Source: three-view drawing plus pictorial views. Frame: mm from the lowest corner of the part. A direction names the side the tool comes from. Give positions to 0.01 mm unless a question says otherwise; leave off trailing zeros. Write each loop counter-clockwise with the first axis right and the second up, starting at its lowest first coordinate (ties: lowest second). Pieces come first, ordered by that corner, then holes.
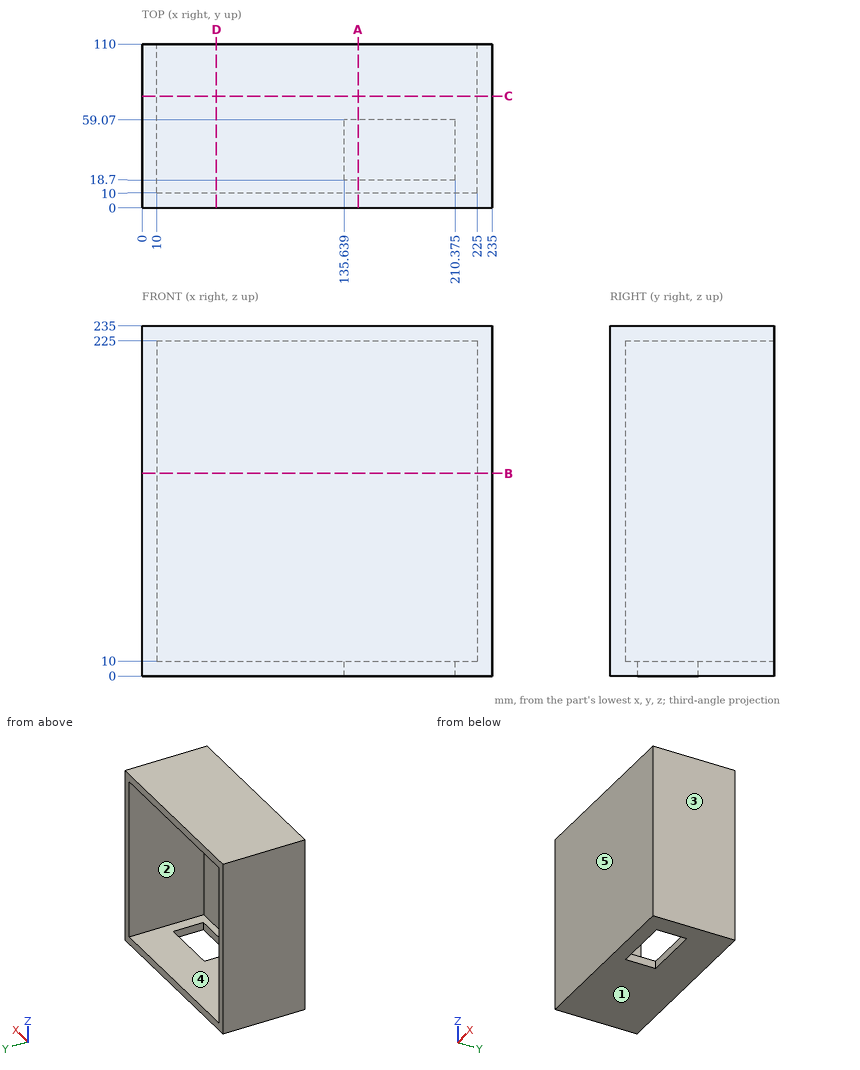
Q1. Section B-B on z = 136. Output: boundary loops of the cut face in (x, y).
Filled sheet:
outline: (0, 0) - (235, 0) - (235, 110) - (225, 110) - (225, 10) - (10, 10) - (10, 110) - (0, 110) - close
Q2. Pin query (flat end, axial travel): P1, Ø4, axis at x = 77, z = 209, coming from the -Y side; P2, Ø8, axis at x = 143, y = 43, coming from the -Z side. Return the tip coordinate at first contact, or that it passes through.
Filled sheet:
P1: stops at y = 0
P2: stops at z = 225
Q3. Section C-C on y = 75. Output: boundary loops of the cut face in (x, z).
Filled sheet:
outline: (0, 0) - (235, 0) - (235, 235) - (0, 235) - close; hole (10, 10) - (225, 10) - (225, 225) - (10, 225) - close
Q4. Section D-D on x = 50. Output: boundary loops of the cut face in (y, z).
Filled sheet:
outline: (0, 0) - (110, 0) - (110, 10) - (10, 10) - (10, 225) - (110, 225) - (110, 235) - (0, 235) - close
Q5. Section A-A on x = 145. Output: boundary loops of the cut face in (y, z).
Filled sheet:
outline: (0, 0) - (18.7, 0) - (18.7, 10) - (10, 10) - (10, 225) - (110, 225) - (110, 235) - (0, 235) - close; (59.07, 0) - (110, 0) - (110, 10) - (59.07, 10) - close
Q6. Access query for the marked faces 4 and 5. Directions: +Z, -Z, +X, -X, +Y, -Y. A direction counts if a zero-diameter tool reaches every point of the face in a straight line with its end or side. Return the directions, or none.
Filled sheet:
face 4: +Y
face 5: +Z, -Z, +X, -X, -Y
Q7. Pull-direction query (Z, two-part tool) for the marked faces 1, 2 and 3; classes: released by +Z, released by -Z, zero draft, split by the parting line, or undercut.
Filled sheet:
face 1: released by -Z
face 2: undercut
face 3: zero draft
Q8. Ray query, line 1 along X through (y, z) = (83.5, 186); line 2 along Y through (x, z) = (98, 23). Return the intervals inside material, ascending.
Filled sheet:
line 1: x = 0 to 10, 225 to 235
line 2: y = 0 to 10
